Geometry: final body of the model. Coordinates: model frame, mm. Face numbers are marked on the shaded views. A direction names the side the tool comes from. Give positions to 0.01 mm unless a question says otherwise; leave off trailing zeros. Write each loop counter-clockwise with the first axis right and the second up, starting at its lowest first coordinate (ties: lowest second). Pieces come first, ordered by that corner, then holes. Notation, with made-up numbers: (21.5, 74) -> (66.5, 74) arc R14 ccw to (66.5, 80) -> close; hole circle Ø9 at (43.25, 29). An arc over 180 degrees is marked (long way). Answer in a Markdown table with one row per item. Add a question column.
from build123d import *

# Parameters (mm, degrees)
SKETCH3_W           = 135.73
SKETCH3_H           = 80.5
BOSS_EXTRUDE1_DEPTH = 5
SKETCH4_W           = 135.73
SKETCH4_H           = 80.5
SKETCH4_W_2         = 125.73
SKETCH4_H_2         = 70.5
BOSS_EXTRUDE2_DEPTH = 45
SKETCH8_W           = 70
SKETCH8_H           = 5
CUT_EXTRUDE2_DEPTH  = 10
DRAFT3_ANGLE        = 21.30578
DRAFT4_ANGLE        = 19.21855
SKETCH12_R          = 1.75
CUT_EXTRUDE3_DEPTH  = 10
CUT_EXTRUDE4_DEPTH  = 45
SKETCH19_R          = 1.6
CUT_EXTRUDE5_DEPTH  = 10
SKETCH20_W          = 50
SKETCH20_H          = 15
CUT_EXTRUDE6_DEPTH  = 15
SKETCH21_R          = 1.5
BOSS_EXTRUDE3_DEPTH = 10


with BuildPart() as part:
    # Sketch3 → Boss-Extrude1 (new body)
    with BuildSketch(Plane(origin=(0, 0, 0), x_dir=(1, 0, 0), z_dir=(0, 1, 0))):
        with Locations((-10.97491424, -60.714595487)):
            Rectangle(SKETCH3_W, SKETCH3_H)
    extrude(amount=BOSS_EXTRUDE1_DEPTH)

    # Sketch4 → Boss-Extrude2 (add)
    with BuildSketch(Plane(origin=(0, 5, 0), x_dir=(1, 0, 0), z_dir=(0, 1, 0))):
        with Locations((-10.97491424, -60.714595487)):
            Rectangle(SKETCH4_W, SKETCH4_H)
        with Locations((-10.97491424, -60.714595487)):
            Rectangle(SKETCH4_W_2, SKETCH4_H_2, mode=Mode.SUBTRACT)
    extrude(amount=BOSS_EXTRUDE2_DEPTH)

    # Sketch8 → Cut-Extrude2 (cut)
    with BuildSketch(Plane(origin=(0, 50, 0), x_dir=(1, 0, 0), z_dir=(0, 1, 0))):
        with Locations((-10.70991424, -98.464595487)):
            Rectangle(SKETCH8_W, SKETCH8_H)
    extrude(amount=-CUT_EXTRUDE2_DEPTH, mode=Mode.SUBTRACT)

    # Draft3
    draft3_faces = [part.faces().sort_by_distance(p)[0] for p in [
        (-10.97491424, 25, 20.464595487),
    ]]
    draft(draft3_faces, Plane(origin=(0, 0, 0), x_dir=(0, 0, -1), z_dir=(0, -1, 0)), DRAFT3_ANGLE)

    # Draft4
    draft4_faces = [part.faces().sort_by_distance(p)[0] for p in [
        (-78.83991424, 25.900276859, 55.664042442),
        (56.89008576, 25.900276859, 55.664042442),
    ]]
    draft(draft4_faces, Plane(origin=(0, 0, 0), x_dir=(0, 0, -1), z_dir=(0, -1, 0)), DRAFT4_ANGLE)

    # Sketch12 → Cut-Extrude3 (cut)
    with BuildSketch(Plane(origin=(0, 0, 95.964595487), x_dir=(-1, 0, 0), z_dir=(0, 0, -1))):
        with Locations((65.83991424, 42)):
            Circle(SKETCH12_R)
        with Locations((65.83991424, 34)):
            Circle(SKETCH12_R)
        with Locations((-43.89008576, 42)):
            Circle(SKETCH12_R)
        with Locations((-43.89008576, 34)):
            Circle(SKETCH12_R)
    extrude(amount=-CUT_EXTRUDE3_DEPTH, mode=Mode.SUBTRACT)

    # Sketch15 → Cut-Extrude4 (cut)
    with BuildSketch(Plane(origin=(0, 50, 0), x_dir=(1, 0, 0), z_dir=(0, 1, 0))):
        Polygon((-73.83991424, -95.964595487), (-75.83991424, -95.964595487), (-75.83991424, -50.577012028), (-75.83991424, -23.464595487), (53.89008576, -23.464595487), (53.89008576, -95.964595487), (51.89008576, -95.964595487), (51.89008576, -25.464595487), (-73.83991424, -25.464595487), align=None)
    extrude(amount=-CUT_EXTRUDE4_DEPTH, mode=Mode.SUBTRACT)

    # Sketch19 → Cut-Extrude5 (cut)
    with BuildSketch(Plane(origin=(0, 5, 0), x_dir=(1, 0, 0), z_dir=(0, 1, 0))):
        with Locations(Location((-45.339914237, -83.561998038, 0), (0, 0, 270))):
            Circle(SKETCH19_R)
        with Locations(Location((-44.06991424, -35.301998038, 0), (0, 0, 270))):
            Circle(SKETCH19_R)
        with Locations(Location((30.86008576, -35.301998033, 0), (0, 0, 270))):
            Circle(SKETCH19_R)
        with Locations(Location((37.210085763, -83.561998033, 0), (0, 0, 270))):
            Circle(SKETCH19_R)
    extrude(amount=-CUT_EXTRUDE5_DEPTH, mode=Mode.SUBTRACT)

    # Sketch20 → Cut-Extrude6 (cut)
    with BuildSketch(Plane(origin=(-70.297258269, -24.505617582, 0), x_dir=(0, 0, 1), z_dir=(-0.9442698473474347, -0.3291723794464724, 0))):
        with Locations((60.964595487, 38.019061203)):
            Rectangle(SKETCH20_W, SKETCH20_H)
    extrude(amount=-CUT_EXTRUDE6_DEPTH, mode=Mode.SUBTRACT)

    # Sketch21 → Boss-Extrude3 (add)
    with BuildSketch(Plane(origin=(0, 50, 0), x_dir=(1, 0, 0), z_dir=(0, 1, 0))):
        with Locations(Location((-65.839914241, -3.464599124, 0), (0, 0, 270))):
            Circle(SKETCH21_R)
        with Locations(Location((43.890085759, -3.464599124, 0), (0, 0, 270))):
            Circle(SKETCH21_R)
    extrude(amount=BOSS_EXTRUDE3_DEPTH)


solid = part.part
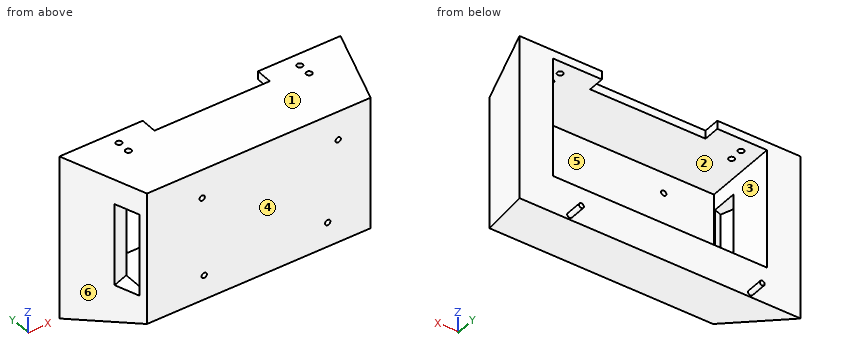
Q1. Access query for the marked faces 1 and 2. Directions: +Z, -Z, +X, -X, +Y, -Y. A direction counts if a zero-diameter tool reaches every point of the face in a straight line with its end or side. Return the directions, or none.
Q2. Contact query for flat-ended pins moving along their axis: pin 1 Ø4 at (x, y) = (37, 42.5) entering from -Z; pin 2 Ø1.5 at (y, z) = (40.5, 55) entering from -X; pin 3 Ø5.5 at (x, y) = (-65.84, 42) entering from -Z; pin 4 Ø1.9 at (x, z) = (-44.07, 35.3) entering from +Y. Output: stop coordinate, or through.
Q3. Line query: probe 1 along Y at (x, z) = (-35, 26); probe 2 along X at (y, z) = (26.5, 30); probe 3 along Z at (x, y) = (51.5, 19.5). Output: solid intervals per line, ascending. Write a range as from..to.
Q4. Section C-C on y = 42. Return loops of the section in (x, z).
Q5. Section B-B on z = 93. Return loops of the section in (x, y), and give its area (3 significant figures).
Q6. Section D-D on x = -35. Return loops of the section in (y, z), and give its area (3 significant figures).
Q7. Section A-A on z = 45. Return loops of the section in (x, y).
Q8. Pull-direction query (X, two-part tool) for the marked faces 3, 4, 5 and 6; classes: +X half, -X half, draft (parallel to the pull), parting line (faces both ways), or undercut.
Checks:
| question | item | result |
|---|---|---|
| 1 | face 1 | +Z, +X, -X, +Y, -Y |
| 1 | face 2 | +Y |
| 2 | pin 1 | z = 3.11 |
| 2 | pin 2 | x = -93.22 |
| 2 | pin 3 | z = 3.01 |
| 2 | pin 4 | through |
| 3 | probe 1 | 0..5 |
| 3 | probe 2 | -88.08..-75.84, 53.89..66.13 |
| 3 | probe 3 | 12.86..23.46, 95.96..100.96 |
| 4 | outline | (-93.48, 4.08) -> (71.53, 4.08) -> (71.53, 100.96) -> (45.64, 100.96) -> (45.64, 95.96) -> (53.89, 95.96) -> (53.89, 23.46) -> (-75.84, 23.46) -> (-75.84, 95.96) -> (-67.59, 95.96) -> (-67.59, 100.96) -> (-93.48, 100.96) -> close; (-64.09, 95.96) -> (-45.71, 95.96) -> (-45.71, 100.96) -> (-64.09, 100.96) -> close; (24.29, 95.96) -> (42.14, 95.96) -> (42.14, 100.96) -> (24.29, 100.96) -> close |
| 5 | outline | (-96.27, 50) -> (-78.84, 0) -> (56.89, 0) -> (74.32, 50) -> (53.89, 50) -> (53.89, 5) -> (-75.84, 5) -> (-75.84, 50) -> close |
| 5 | area | 1,820 mm^2 |
| 6 | outline | (0, 20.46) -> (50, 0.96) -> (50, 23.46) -> (5, 23.46) -> (5, 95.96) -> (40, 95.96) -> (40, 100.96) -> (0, 100.96) -> close |
| 6 | area | 1,200 mm^2 |
| 7 | outline | (-96.27, 50) -> (-85.28, 18.48) -> (-75.84, 21.77) -> (-75.84, 50) -> close; (-80.34, 4.31) -> (-78.84, 0) -> (56.89, 0) -> (74.32, 50) -> (53.89, 50) -> (53.89, 5) -> (-75.84, 5) -> (-75.84, 5.88) -> close |
| 8 | face 3 | undercut |
| 8 | face 4 | draft |
| 8 | face 5 | undercut |
| 8 | face 6 | -X half |
